Read the model definition and answer for the solid it produces. Units are mm, in the model's axes. Coordinates: 2 decimals unless noted, no trailing zeros. Loops run counter-clockwise (first coordinate to the right, second up) from the corner with the lowest first, then second, coordinate; pieces in that order, holes last.
from build123d import *

# Parameters (mm, degrees)
F0_W     = 38.1
F0_H     = 19.05
F1_DEPTH = 558.8
F2_R     = 5.08


with BuildPart() as f1:
    # F0 (on Right) → F1 (new body, symmetric)
    with BuildSketch(Plane.YZ):
        Rectangle(F0_W, F0_H)
    extrude(amount=F1_DEPTH, both=True)

    # F2
    f2_edges = [f1.edges().sort_by_distance(p)[0] for p in [
        (0, -19.05, 9.525),
        (0, -19.05, -9.525),
        (0, 19.05, 9.525),
        (0, 19.05, -9.525),
    ]]
    fillet(f2_edges, radius=F2_R)


solid = f1.part
Item 1: A cutting plane is placed at A-A on x = -401.5. Determine the outline of the cut face in (y, z) (3 decimals).
Numbers:
outline: (-19.05, -4.445) arc R5.08 ccw to (-13.97, -9.525) - (13.97, -9.525) arc R5.08 ccw to (19.05, -4.445) - (19.05, 4.445) arc R5.08 ccw to (13.97, 9.525) - (-13.97, 9.525) arc R5.08 ccw to (-19.05, 4.445) - close
Item 2: Given pin 1 (1 mm diameter, centred on x = -262, z = 5.5, fed in from -Y), flat-ended and moving along its own axis, determine where the tip first touches the part or whether it passes through.
Numbers:
pin 1: stops at y = -19.02
Item 3: Find the intervals of material crossed by line 1 along Z through (x, y) = (131.5, -15); line 2 along Y through (x, z) = (348, -5); line 3 along Z through (x, y) = (175, 14.5), in increasing order.
Numbers:
line 1: z = -9.42 to 9.42
line 2: y = -19.02 to 19.02
line 3: z = -9.5 to 9.5
